For this review, take the finished solid that the model builds, in its own axes (mm). Face numbers are marked on the shaded views. Coordinates: 2 decimals unless noted, no trailing zeros. Write each loop counter-clockwise with the first axis right and the second up, starting at its lowest first coordinate (ties: lowest second). Pieces come first, ordered by that corner, then holes.
```python
from build123d import *

# Parameters (mm, degrees)
ESQUISSE1_R                     = 38.550000000000004
ESQUISSE1_R_2                   = 26.55
BOSS_EXTRU_1_DEPTH              = 50
TROU_TARAUD_M4X0_71_D           = 3.3
TROU_TARAUD_M4X0_71_DEPTH       = 16
TROU_TARAUD_M4X0_71_CSINK_D     = 4.05
TROU_TARAUD_M4X0_71_CSINK_ANGLE = 90
TROU_TARAUD_M4X0_71_TIP         = 0.9914200213954745


# Read off the part's stored shape, not the designer's step: Trou taraudé M4x0.74
with BuildPart() as part:
    # Esquisse1 → Boss.-Extru.1 (new body)
    with BuildSketch(Plane(origin=(0, 0, 0), x_dir=(1, 0, 0), z_dir=(0, 1, 0))):
        with Locations(Location((0, 0, 0), (0, 0, 270))):
            Circle(ESQUISSE1_R)
        with Locations(Location((0, 0, 0), (0, 0, 270))):
            Circle(ESQUISSE1_R_2, mode=Mode.SUBTRACT)
    extrude(amount=BOSS_EXTRU_1_DEPTH)

    # Trou taraudé M4x0.71
    with Locations(Plane(origin=(0, 0, 0), x_dir=(-1, 0, 0), z_dir=(0, -1, 0))):
        with Locations((-23.016325728, -23.016325728), (-23.016325728, 23.016325728), (23.016325728, 23.016325728), (23.016325728, -23.016325728)):
            CounterSinkHole(TROU_TARAUD_M4X0_71_D / 2, TROU_TARAUD_M4X0_71_CSINK_D / 2, depth=TROU_TARAUD_M4X0_71_DEPTH, counter_sink_angle=TROU_TARAUD_M4X0_71_CSINK_ANGLE)
            with Locations((0, 0, -(TROU_TARAUD_M4X0_71_DEPTH + TROU_TARAUD_M4X0_71_TIP / 2))):  # 118° drill point
                Cone(0, TROU_TARAUD_M4X0_71_D / 2, TROU_TARAUD_M4X0_71_TIP, mode=Mode.SUBTRACT)

    # Trou taraudé M4x0.74 outline → Trou taraudé M4x0.74 (revolve, cut)
    with BuildSketch(Plane(origin=(0, 39.944411858, 0), x_dir=(0.4998061049474771, 0, -0.8661373202080785), z_dir=(0, -1, 0))):
        Polygon((0, -38.55002295), (2.02502295, -38.55002295), (1.65, -38.175), (1.65, -26.498651577), (0, -26.498651577), align=None)
    revolve(axis=Axis((0, 39.944411858, 0), (0.8661373202080785, 0, 0.4998061049474771)), mode=Mode.SUBTRACT)

    # Trou taraud_ M4x0.74 2 outline → Trou taraud_ M4x0.74 2 (revolve, cut)
    with BuildSketch(Plane(origin=(0, 40.055300006, 0), x_dir=(0.49980598723152586, 0, 0.8661373881362702), z_dir=(0, 1.0000000000000002, 0))):
        Polygon((2.025014074, 38.550014074), (0, 38.550014074), (0, 26.498651577), (1.65, 26.498651577), (1.65, 38.175), align=None)
    revolve(axis=Axis((0, 40.055300006, 0), (0.8661373881362704, 0, -0.49980598723152597)), mode=Mode.SUBTRACT)

    # Trou taraud_ M4x0.74 3 outline → Trou taraud_ M4x0.74 3 (revolve, cut)
    with BuildSketch(Plane(origin=(0, 40.043688013, 0), x_dir=(0.9999999999344692, 0, 1.1448216284808903e-05), z_dir=(0, 1, 0))):
        Polygon((0, -38.549999963), (2.024999963, -38.549999963), (1.65, -38.175), (1.65, -26.498658226), (0, -26.498658226), align=None)
    revolve(axis=Axis((0, 40.043688013, 0), (1.1448216284808903e-05, 0, -0.9999999999344692)), mode=Mode.SUBTRACT)


solid = part.part
```
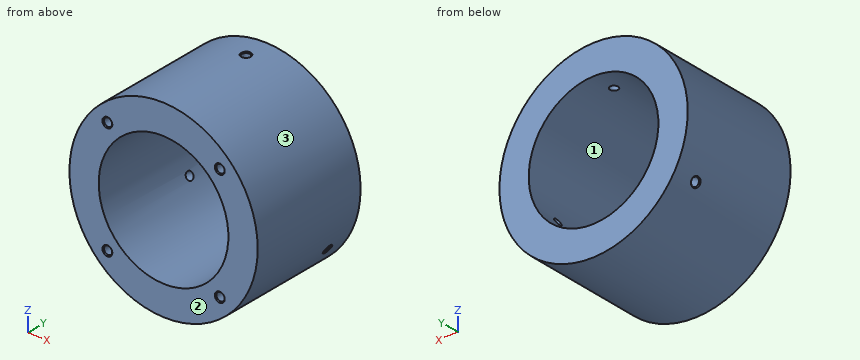
1) Consider section B-B (x = -13). Give the boundary of the cut face in (y, z), then the cut area to 3 significant figures.
2) Clearance check with flat-ended pins moving along their axes: P1, Ø12, axis at y = 40, z = -10.5, coming from the +X side; P2, Ø2, axis at y = 36.5, z = -17.5, coming from the -X side; P3, Ø1.5, axis at y = 39.5, z = -6.5, coming from the +X side. State where each tip first meets the part, or that it passes through.
3) Consider section A-A (z = 0). Give the boundary of the cut face in (x, y).
4) Consider section C-C (y = 6). Give the boundary of the cut face in (x, z).
5) Consider section D-D (y = 26.5). Give the boundary of the cut face in (x, z), then the cut area to 3 significant figures.
6) The part is to be moulded in two halves that separate along X. For the marked faces 1, 2 and 3, say which applies: pulls with the +X half, pulls with the -X half, needs draft (parallel to the pull), parting line crosses it, or undercut.
7) For L1, parallel to X at y = 47, z = 1; L2, parallel to Z at x = -22, y = 7; L3, parallel to Z at x = -17.5, y = 14.5, list the stretches that pass through material, from the lowest coordinate up.
Results:
1. outline: (0, -36.29) - (50, -36.29) - (50, -23.15) - (0, -23.15) - close; (0, 23.15) - (50, 23.15) - (50, 36.29) - (0, 36.29) - close
1. area: 1,310 mm2
2. P1: stops at x = 38.29
2. P2: stops at x = -34.84
2. P3: stops at x = 38.12
3. outline: (-38.55, 0) - (-26.55, 0) - (-26.55, 50) - (-38.55, 50) - close; (26.55, 0) - (38.55, 0) - (38.55, 50) - (26.55, 50) - close
4. outline: circle Ø77.1 at (0, 0); hole circle Ø53.1 at (0, 0); hole circle Ø3.3 at (-23.02, -23.02); hole circle Ø3.3 at (-23.02, 23.02); hole circle Ø3.3 at (23.02, -23.02); hole circle Ø3.3 at (23.02, 23.02)
5. outline: circle Ø77.1 at (0, 0); hole circle Ø53.1 at (0, 0)
5. area: 2,450 mm2
6. face 1: undercut
6. face 2: needs draft
6. face 3: parting line crosses it
7. L1: x = -38.54 to -26.53, 26.53 to 38.54
7. L2: z = -31.66 to -24.32, -21.72 to -14.86, 14.86 to 21.72, 24.32 to 31.66
7. L3: z = -34.35 to -19.97, 19.97 to 34.35
